from build123d import *

# Parameters (mm, degrees)
Y_KSEKLIK_EKSTR_ZYON3_DEPTH = 25
Y_KSEKLIK_EKSTR_ZYON4_DEPTH = 15
IZIM11_R                    = 3.5
KES_EKSTR_ZYON3_DEPTH       = 10
KES_EKSTR_ZYON4_DEPTH       = 16
KES_EKSTR_ZYON5_REACH       = 77.444


with BuildPart() as part:
    # Çizim6 → Yükseklik-Ekstrüzyon3 (new, symmetric)
    with BuildSketch(Plane.XY):
        with BuildLine():
            Line((-119.371512251, 18.973770729), (-115.371512251, 18.973770729))
            Line((-115.371512251, 18.973770729), (-110.371512251, 18.973770729))
            Line((-110.371512251, 18.973770729), (-110.371512251, 20.773770729))
            Line((-110.371512251, 20.773770729), (-110.371512251, 26.023770729))
            ThreePointArc((-110.371512251, 26.023770729), (-111.92384631, 29.771436669), (-115.671512251, 31.323770729))
            Line((-115.671512251, 31.323770729), (-120.921512251, 31.323770729))
            Line((-120.921512251, 31.323770729), (-122.721512251, 31.323770729))
            Line((-122.721512251, 31.323770729), (-128.221512251, 31.323770729))
            Line((-128.221512251, 31.323770729), (-130.021512251, 31.323770729))
            Line((-130.021512251, 31.323770729), (-135.271512251, 31.323770729))
            ThreePointArc((-135.271512251, 31.323770729), (-139.019178191, 29.771436669), (-140.571512251, 26.023770729))
            Line((-140.571512251, 26.023770729), (-140.571512251, 20.773770729))
            Line((-140.571512251, 20.773770729), (-140.571512251, 16.223770729))
            Line((-140.571512251, 16.223770729), (-140.571512251, 11.673770729))
            Line((-140.571512251, 11.673770729), (-140.571512251, 6.423770729))
            ThreePointArc((-140.571512251, 6.423770729), (-139.019178191, 2.676104789), (-135.271512251, 1.123770729))
            Line((-135.271512251, 1.123770729), (-130.021512251, 1.123770729))
            Line((-130.021512251, 1.123770729), (-128.221512251, 1.123770729))
            Line((-128.221512251, 1.123770729), (-128.221512251, 6.123770729))
            Line((-128.221512251, 6.123770729), (-128.221512251, 10.123770729))
            Line((-128.221512251, 10.123770729), (-122.721512251, 10.123770729))
            Line((-122.721512251, 10.123770729), (-122.721512251, 6.123770729))
            Line((-122.721512251, 6.123770729), (-122.721512251, 1.123770729))
            Line((-122.721512251, 1.123770729), (-120.921512251, 1.123770729))
            Line((-120.921512251, 1.123770729), (-115.671512251, 1.123770729))
            ThreePointArc((-115.671512251, 1.123770729), (-111.92384631, 2.676104789), (-110.371512251, 6.423770729))
            Line((-110.371512251, 6.423770729), (-110.371512251, 11.673770729))
            Line((-110.371512251, 11.673770729), (-110.371512251, 13.473770729))
            Line((-110.371512251, 13.473770729), (-115.371512251, 13.473770729))
            Line((-115.371512251, 13.473770729), (-119.371512251, 13.473770729))
            Line((-119.371512251, 13.473770729), (-119.371512251, 18.973770729))
        make_face()
        with BuildLine():
            Line((-133.871512251, 20.323770729), (-135.071512251, 20.323770729))
            Line((-135.071512251, 20.323770729), (-135.871512251, 20.323770729))
            Line((-135.871512251, 20.323770729), (-135.971512251, 20.323770729))
            Line((-135.971512251, 20.323770729), (-135.971512251, 26.723770729))
            Line((-135.971512251, 26.723770729), (-129.571512251, 26.723770729))
            Line((-129.571512251, 26.723770729), (-129.571512251, 26.623770729))
            Line((-129.571512251, 26.623770729), (-129.571512251, 25.823770729))
            Line((-129.571512251, 25.823770729), (-129.571512251, 24.623770729))
            ThreePointArc((-129.571512251, 24.623770729), (-129.659380216, 24.411638694), (-129.871512251, 24.323770729))
            Line((-129.871512251, 24.323770729), (-130.921512251, 24.323770729))
            ThreePointArc((-130.921512251, 24.323770729), (-130.992222929, 24.294481407), (-131.021512251, 24.223770729))
            Line((-131.021512251, 24.223770729), (-131.021512251, 23.056613441))
            ThreePointArc((-131.021512251, 23.056613441), (-131.013900204, 23.018345098), (-130.992222929, 22.985902763))
            Line((-130.992222929, 22.985902763), (-128.359380216, 20.353060051))
            ThreePointArc((-128.359380216, 20.353060051), (-128.326937882, 20.331382776), (-128.288669538, 20.323770729))
            Line((-128.288669538, 20.323770729), (-122.654354963, 20.323770729))
            ThreePointArc((-122.654354963, 20.323770729), (-122.61608662, 20.331382776), (-122.583644285, 20.353060051))
            Line((-122.583644285, 20.353060051), (-119.950801573, 22.985902763))
            ThreePointArc((-119.950801573, 22.985902763), (-119.929124298, 23.018345098), (-119.921512251, 23.056613441))
            Line((-119.921512251, 23.056613441), (-119.921512251, 24.223770729))
            ThreePointArc((-119.921512251, 24.223770729), (-119.950801573, 24.294481407), (-120.021512251, 24.323770729))
            Line((-120.021512251, 24.323770729), (-121.071512251, 24.323770729))
            ThreePointArc((-121.071512251, 24.323770729), (-121.283644285, 24.411638694), (-121.371512251, 24.623770729))
            Line((-121.371512251, 24.623770729), (-121.371512251, 25.823770729))
            Line((-121.371512251, 25.823770729), (-121.371512251, 26.323770729))
            Line((-121.371512251, 26.323770729), (-121.371512251, 26.723770729))
            Line((-121.371512251, 26.723770729), (-114.971512251, 26.723770729))
            Line((-114.971512251, 26.723770729), (-114.971512251, 20.323770729))
            Line((-114.971512251, 20.323770729), (-115.371512251, 20.323770729))
            Line((-115.371512251, 20.323770729), (-115.871512251, 20.323770729))
            Line((-115.871512251, 20.323770729), (-117.071512251, 20.323770729))
            ThreePointArc((-117.071512251, 20.323770729), (-117.283644285, 20.411638694), (-117.371512251, 20.623770729))
            Line((-117.371512251, 20.623770729), (-117.371512251, 21.673770729))
            ThreePointArc((-117.371512251, 21.673770729), (-117.400801573, 21.744481407), (-117.471512251, 21.773770729))
            Line((-117.471512251, 21.773770729), (-118.638669538, 21.773770729))
            ThreePointArc((-118.638669538, 21.773770729), (-118.676937882, 21.766158682), (-118.709380216, 21.744481407))
            Line((-118.709380216, 21.744481407), (-121.342222929, 19.111638694))
            ThreePointArc((-121.342222929, 19.111638694), (-121.363900204, 19.07919636), (-121.371512251, 19.040928016))
            Line((-121.371512251, 19.040928016), (-121.371512251, 13.406613441))
            ThreePointArc((-121.371512251, 13.406613441), (-121.363900204, 13.368345098), (-121.342222929, 13.335902763))
            Line((-121.342222929, 13.335902763), (-118.709380216, 10.703060051))
            ThreePointArc((-118.709380216, 10.703060051), (-118.676937882, 10.681382776), (-118.638669538, 10.673770729))
            Line((-118.638669538, 10.673770729), (-117.471512251, 10.673770729))
            ThreePointArc((-117.471512251, 10.673770729), (-117.400801573, 10.703060051), (-117.371512251, 10.773770729))
            Line((-117.371512251, 10.773770729), (-117.371512251, 11.823770729))
            ThreePointArc((-117.371512251, 11.823770729), (-117.283644285, 12.035902763), (-117.071512251, 12.123770729))
            Line((-117.071512251, 12.123770729), (-115.871512251, 12.123770729))
            Line((-115.871512251, 12.123770729), (-115.371512251, 12.123770729))
            Line((-115.371512251, 12.123770729), (-114.971512251, 12.123770729))
            Line((-114.971512251, 12.123770729), (-114.971512251, 5.723770729))
            Line((-114.971512251, 5.723770729), (-121.371512251, 5.723770729))
            Line((-121.371512251, 5.723770729), (-121.371512251, 6.123770729))
            Line((-121.371512251, 6.123770729), (-121.371512251, 6.623770729))
            Line((-121.371512251, 6.623770729), (-121.371512251, 7.823770729))
            ThreePointArc((-121.371512251, 7.823770729), (-121.283644285, 8.035902763), (-121.071512251, 8.123770729))
            Line((-121.071512251, 8.123770729), (-120.021512251, 8.123770729))
            ThreePointArc((-120.021512251, 8.123770729), (-119.950801573, 8.153060051), (-119.921512251, 8.223770729))
            Line((-119.921512251, 8.223770729), (-119.921512251, 9.390928016))
            ThreePointArc((-119.921512251, 9.390928016), (-119.929124298, 9.42919636), (-119.950801573, 9.461638694))
            Line((-119.950801573, 9.461638694), (-122.583644285, 12.094481407))
            ThreePointArc((-122.583644285, 12.094481407), (-122.61608662, 12.116158682), (-122.654354963, 12.123770729))
            Line((-122.654354963, 12.123770729), (-128.288669538, 12.123770729))
            ThreePointArc((-128.288669538, 12.123770729), (-128.326937882, 12.116158682), (-128.359380216, 12.094481407))
            Line((-128.359380216, 12.094481407), (-130.992222929, 9.461638694))
            ThreePointArc((-130.992222929, 9.461638694), (-131.013900204, 9.42919636), (-131.021512251, 9.390928016))
            Line((-131.021512251, 9.390928016), (-131.021512251, 8.223770729))
            ThreePointArc((-131.021512251, 8.223770729), (-130.992222929, 8.153060051), (-130.921512251, 8.123770729))
            Line((-130.921512251, 8.123770729), (-129.871512251, 8.123770729))
            ThreePointArc((-129.871512251, 8.123770729), (-129.659380216, 8.035902763), (-129.571512251, 7.823770729))
            Line((-129.571512251, 7.823770729), (-129.571512251, 6.623770729))
            Line((-129.571512251, 6.623770729), (-129.571512251, 6.123770729))
            Line((-129.571512251, 6.123770729), (-129.571512251, 5.723770729))
            Line((-129.571512251, 5.723770729), (-135.971512251, 5.723770729))
            Line((-135.971512251, 5.723770729), (-135.971512251, 12.123770729))
            Line((-135.971512251, 12.123770729), (-135.571512251, 12.123770729))
            Line((-135.571512251, 12.123770729), (-135.071512251, 12.123770729))
            Line((-135.071512251, 12.123770729), (-133.871512251, 12.123770729))
            ThreePointArc((-133.871512251, 12.123770729), (-133.659380216, 12.035902763), (-133.571512251, 11.823770729))
            Line((-133.571512251, 11.823770729), (-133.571512251, 10.773770729))
            ThreePointArc((-133.571512251, 10.773770729), (-133.542222929, 10.703060051), (-133.471512251, 10.673770729))
            Line((-133.471512251, 10.673770729), (-132.304354963, 10.673770729))
            ThreePointArc((-132.304354963, 10.673770729), (-132.26608662, 10.681382776), (-132.233644285, 10.703060051))
            Line((-132.233644285, 10.703060051), (-129.600801573, 13.335902763))
            ThreePointArc((-129.600801573, 13.335902763), (-129.579124298, 13.368345098), (-129.571512251, 13.406613441))
            Line((-129.571512251, 13.406613441), (-129.571512251, 19.040928016))
            ThreePointArc((-129.571512251, 19.040928016), (-129.579124298, 19.07919636), (-129.600801573, 19.111638694))
            Line((-129.600801573, 19.111638694), (-132.233644285, 21.744481407))
            ThreePointArc((-132.233644285, 21.744481407), (-132.26608662, 21.766158682), (-132.304354963, 21.773770729))
            Line((-132.304354963, 21.773770729), (-133.471512251, 21.773770729))
            ThreePointArc((-133.471512251, 21.773770729), (-133.542222929, 21.744481407), (-133.571512251, 21.673770729))
            Line((-133.571512251, 21.673770729), (-133.571512251, 20.623770729))
            ThreePointArc((-133.571512251, 20.623770729), (-133.659380216, 20.411638694), (-133.871512251, 20.323770729))
        make_face(mode=Mode.SUBTRACT)
    extrude(amount=Y_KSEKLIK_EKSTR_ZYON3_DEPTH, both=True)

    # Çizim8 → Yükseklik-Ekstrüzyon4 (add)
    with BuildSketch(Plane.ZY.offset(140.571512251)):
        Polygon((31.764979794, -6.075019791), (-16.444090932, 51.378313443), (-31.764979794, 38.522561249), (16.444090932, -18.930771985), align=None)
    extrude(amount=Y_KSEKLIK_EKSTR_ZYON4_DEPTH)

    # Çizim11 → Kes-Ekstrüzyon3 (cut)
    with BuildSketch(Plane.ZY.offset(155.571512251)):
        with Locations(Location((17.998053071, -5.225473678, 0), (0, 0, 270))):
            Circle(IZIM11_R)
        with Locations(Location((-17.998053071, 37.673015136, 0), (0, 0, 270))):
            Circle(IZIM11_R)
    extrude(amount=-KES_EKSTR_ZYON3_DEPTH, mode=Mode.SUBTRACT)

    # Çizim12 → Kes-Ekstrüzyon4 (cut)
    with BuildSketch(Plane(origin=(0, 13.13114735, 15.64909203), x_dir=(1, 0, 0), z_dir=(-3.3982743057988955e-15, 0.6427876096865416, 0.7660444431189761))):
        Polygon((-142.571512251, 47.928129413), (-153.571512251, 47.928129413), (-153.571512251, 36.149140278), (-153.571512251, -23.071870587), (-142.571512251, -23.071870587), (-142.571512251, -8.755858334), (-142.571512251, 16.830124537), align=None)
    extrude(amount=-KES_EKSTR_ZYON4_DEPTH, mode=Mode.SUBTRACT)

    # Kes-Ekstrüzyon5: up to this face of the body (flat: up to its plane)
    kes_ekstr_zyon5_end = Plane(part.part.faces().sort_by_distance((-142.571512251, 17.509345948, 1.532088886))[0])
    # Çizim13 → Kes-Ekstrüzyon5 (cut, up to the picked face)
    with BuildSketch(Plane.ZY.offset(155.571512251), mode=Mode.PRIVATE) as kes_ekstr_zyon5_sk1:
        Polygon((-5.838095372, 38.738580131), (-21.158984235, 25.882827937), (5.838095372, -6.291038674), (21.158984235, 6.56471352), align=None)
    kes_ekstr_zyon5_tool1 = split(extrude(kes_ekstr_zyon5_sk1.sketch, amount=-KES_EKSTR_ZYON5_REACH, mode=Mode.PRIVATE), bisect_by=kes_ekstr_zyon5_end, keep=Keep.BOTH, mode=Mode.PRIVATE)
    add(kes_ekstr_zyon5_tool1.solids().sort_by(Axis((-155.571512, 16.223771, 0), (1, 0, 0)))[0], mode=Mode.SUBTRACT)


solid = part.part
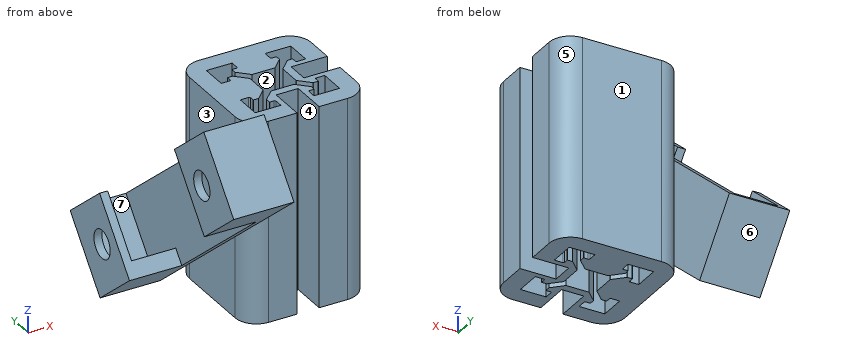
CAD build for the part. Positions are in the model's coordinates, mm. Face numbers are marked on the shaded views. A direction names the side the tool comes from. Coordinates: 2 decimals unless noted, no trailing zeros. Write each loop counter-clockwise with the first axis right and the second up, starting at its lowest first coordinate (ties: lowest second). Pieces come first, ordered by that corner, then holes. Notation, with made-up numbers: M 2.5,-34.75 L 42.5,-34.75 A14 cw 42.5,-24.75 Z; hole C -30.75,29.5 d2. An arc over 180 degrees is marked long. Answer as a JSON object with one key per item and string values. Group by question number.
1) Saw through at B-B (y = -7.5). Write the cut outline in (x, z), plus the area to 3 significant figures.
2) Mould opens along X. For the marked faces 5, 6 and 7 say: +X half, -X half, draft (parallel to the pull), parting line (faces both ways), or undercut.
3) Pin check, flat tips, straight feed: pin 1 Ø0.9 at (x, z) = (-132.5, 4.5) entering from +Y; pin 2 Ø2.5 at (x, z) = (-116.5, -11) entering from -Y; pin 3 Ø6.5 at (y, z) = (40.5, -19) entering from +X. Stop position of each tip, or through.
4) Wall check: line 1 (X direction, y = 9, z = 16); line 2 (X direction, y = 23, z = -18.5); line 3 (Y direction, x = -132.5, z = 3.5). Give the ranges that are in metal, low to high. Write a range as from..to.
5) Saw through at A-A (z = -9). Give the number of separate pieces and of enclosed holes in the cut face, plus the area to 3 significant figures.
6) Tool access for the marked faces 1, 2, 3 and 4: list every direction of +Z, -Z, +X, -X, +Y, -Y with a clear straight run to the whole face (end or side of a thin tool).
Values follow:
{
 "1": {"outline": "M -155.57,6.85 L -140.57,6.85 L -140.57,30.07 L -155.57,30.07 L -155.57,20.66 L -153.57,20.66 L -153.57,26.96 L -142.57,26.96 L -142.57,12.07 L -153.57,12.07 L -153.57,15.34 L -155.57,15.34 Z", "area": "174 mm2"},
 "2": {"face 5": "+X half", "face 6": "draft", "face 7": "undercut"},
 "3": {"pin 1": "stops at y = 31.32", "pin 2": "stops at y = 1.12", "pin 3": "stops at x = -140.57"},
 "4": {"line 1": "x = -142.57..-135.97, -131.02..-128.22, -122.72..-119.92, -114.97..-110.37", "line 2": "x = -142.57..-135.97, -131..-119.94, -114.97..-110.37", "line 3": "y = 1.12..5.72, 10.67..21.77, 26.72..31.32"},
 "5": {"separate pieces": "2", "enclosed holes": "1", "area": "650 mm2"},
 "6": {"face 1": "+Z, -Z, +X, +Y", "face 2": "+Z, -Z", "face 3": "+Z, -X, +Y", "face 4": "+Z, -Z, -Y"}
}
